Geometry: final body of the model. Coordinates: model frame, mm. A direction names the side the tool comes from. Give positions to 0.01 mm unless a question says otherwise; leave off trailing zeros. Write each loop counter-clockwise with the first axis right and the second up, starting at its lowest first coordinate (ties: lowest second). Pieces come first, ordered by that corner, then holes. Notation, with made-up numbers: M -9,72.5 L 25,72.5 A24 cw 25,110.5 Z; hole C 15.25,-32 d7. An arc over 180 degrees is marked long. One line per question, with ' | ' between items.
Autodesk Inventor part; units mm, degrees
ref_plane "YZ Plane" through (0, 0, 0) normal (1, 0, 0) x (0, 1, 0)
ref_plane "XZ Plane" through (0, 0, 0) normal (0, 1, 0) x (-1, 0, 0)
ref_plane "XY Plane" through (0, 0, 0) normal (0, 0, 1) x (1, 0, 0)
ref_plane "Work Plane1" through (0, 0, 0) normal (0, 0, 1) x (1, 0, 0)
sketch "Sketch1" plane through (0, 0, 0) normal (0, 0, 1) x (1, 0, 0)
  circle A0 centre (15, -11) radius 1.5
  circle A1 centre (30, -11) radius 1.5
  line L0 (0, -20) -> (0, 4) construction
  line L1 (0, -20) -> (45, -20) construction
  line L2 (45, -20) -> (45, 4) construction
  line L3 (0, 4) -> (45, 4) construction
  line L4 (15, -11) -> (10, -11) construction
  line L5 (10, -11) -> (10, -6) construction
  line L6 (10, -6) -> (15, -6) construction
  line L7 (15, -6) -> (15, -11) construction
  line L8 (30, -11) -> (35, -11) construction
  line L9 (35, -11) -> (35, -6) construction
  line L10 (35, -6) -> (30, -6) construction
  line L11 (30, -6) -> (30, -11) construction
  line L12 (10, -6) -> (35, -6)
  line L13 (35, -6) -> (35, -16)
  line L14 (35, -16) -> (10, -16)
  line L15 (10, -16) -> (10, -6)
  line L16 (22.5, -16) -> (-7.5, -16)
  line L17 (-7.5, -16) -> (52.5, -16)
  line L18 (52.5, -16) -> (52.5, -46)
  line L19 (52.5, -46) -> (-7.5, -46)
  line L20 (-7.5, -46) -> (-7.5, -16)
  point P0 (0, 0)
  dimension "d0" = 5
  dimension "d1" = 5
  dimension "d2" = 5
  dimension "d3" = 5
  dimension "d4" = 10
  dimension "d5" = 30
  dimension "d6" = 60
  dimension "d7" = 30
extrude "Extrusion1" add sketch "Sketch1" along normal blind 2
properties part number "april_tag_2"
(1) Set-up query: faces 4 (the face through (1, -16, 1)), 5 (the face through (35, -11, 1)), 6 (the face through (-7.5, -31, 1)). Return all of +Z, -Z, +X, -X, +Y, -Y with unobstructed straight access to the full face (end or side cutting, diameter ignored); none if empty.
Working result:
face 4: +Z, -Z, -X, +Y | face 5: +Z, -Z, +X, +Y | face 6: +Z, -Z, -X, +Y, -Y
(2) Cut plane B-B, the plane x = 15. Return loops of the section in (y, z), then the cut area to 3 significant figures.
Working result:
outline: M -46,0 L -12.5,0 L -12.5,2 L -46,2 Z; M -9.5,0 L -6,0 L -6,2 L -9.5,2 Z | area: 74.0 mm^2
(3) Cut plane A-A, the plane y = -11. Return loops of the section in (x, z).
Working result:
outline: M 10,0 L 13.5,0 L 13.5,2 L 10,2 Z; M 16.5,0 L 28.5,0 L 28.5,2 L 16.5,2 Z; M 31.5,0 L 35,0 L 35,2 L 31.5,2 Z
(4) Material intervals for L1, parallel to Y at x = 30, z = 0.95; L2, parallel to X at y = -14, z = 0.25; L3, parallel to Y at x = 49.5, z = 1.9, sorted ascending. Write a range as [from, to].
Working result:
L1: y = [-46, -12.5], [-9.5, -6] | L2: x = [10, 35] | L3: y = [-46, -16]
(5) Cut plane D-D, the plane x = 45.5. Return loops of the section in (y, z), then the cut area to 3 significant figures.
Working result:
outline: M -46,0 L -16,0 L -16,2 L -46,2 Z | area: 60.0 mm^2
(6) Cut plane C-C, the plane z = 0.55. Return loops of the section in (x, y), then the cut area to 3 significant figures.
Working result:
outline: M -7.5,-46 L 52.5,-46 L 52.5,-16 L 35,-16 L 35,-6 L 10,-6 L 10,-16 L -7.5,-16 Z; hole C 15,-11 d3; hole C 30,-11 d3 | area: 2,040 mm^2
(7) Draft query along X for faces 1 (the face through (22, -6, 1)), 2 (the face through (28.5, -11.07, 0.99)), 3 (the face through (10, -11, 1)). Return one class per face: released by +X, released by -X, zero draft, split by the parting line, or undercut.
Working result:
face 1: zero draft | face 2: undercut | face 3: released by -X
(8) First-contact query: P1, Ø1, axis at x = 44, y = -16.5, coming from the -Z side; P2, Ø0.6, axis at x = 45.5, z = 1.5, coming from the +Y side. Flat tips, straight axial feed; report the tip coordinate or a pass-through.
Working result:
P1: stops at z = 0 | P2: stops at y = -16
